The drawing under review shows one solid part. Ordinate dimensions are in mm from its lowest x, y, z. A direction names the side the tool comes from. Give positions to 0.01 mm unless a question says otherwise; leave off trailing zeros. Order: outer loops, then holes, each group sorted by start corner. A loop starts at its lowest first (then second) coordinate and runs counter-clockwise, first axis right, second up. Notation, with made-up numbers: (-22.75, -15) - (13.25, -15) arc R8 ccw to (13.25, -2) - close; hole circle Ø1 at (-36.75, 11.5). An arc over 180 degrees is marked (long way). Use CSV: the item, a comma, the result in double quotes. Start each with the question number.
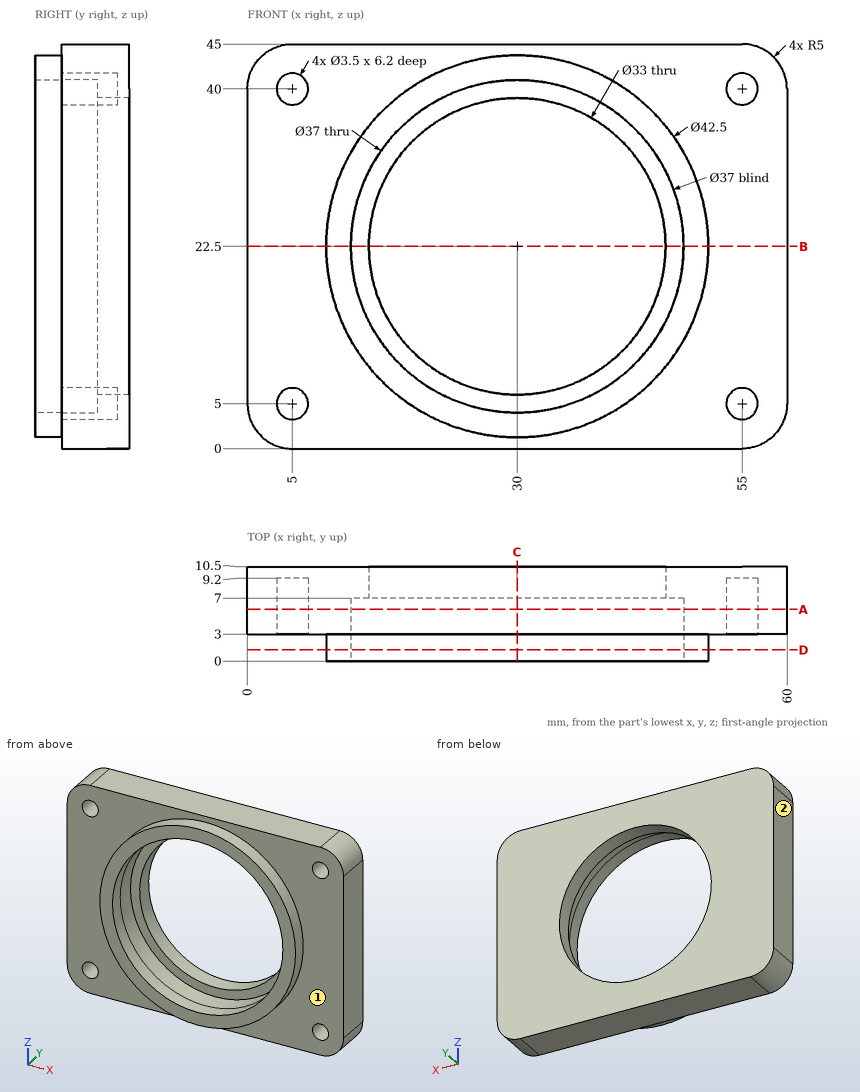
1. Consider section C-C (x = 30). Give the boundary of the cut face in (y, z).
2. To check wall thickness, follow L1, parallel to Z at x = 54, y = 7.5; L2, parallel to X at y = 5.55, z = 22.5; L3, parallel to Z at x = 30, y = 4.15. State the ranges of each line that lie inside material, in increasing order. Write a range as [from, to].
3. Clearance check with flat-ended pins moving along their axes: pin 1 (4 mm diameter, centred on y = 5.5, z = 11.5, fed in from -X); pin 2 (1.8 mm diameter, centred on x = 54, z = 40.5, fed in from -Y); pin 3 (2 mm diameter, centred on x = 55, z = 40, fed in from -Y); pin 4 (22 mm diameter, centred on x = 30, z = 22.5, fed in from -Y). State where each tip first meets the part, or that it passes through.
4. Consider section A-A (y = 5.75). Give the boundary of the cut face in (x, z), and give its area (3 significant figures).
5. Tool access review of the marked faces 1 and 2: name each direction out of +Z, -Z, +X, -X, +Y, -Y from which nothing blocks a thin tool from reaching the whole face with its end or side.
6. Consider section B-B (z = 22.5). Give the boundary of the cut face in (x, y).
7. Consider section D-D (y = 1.25). Give the boundary of the cut face in (x, z).
Answers follow:
1,outline,"(0, 1.25) - (3, 1.25) - (3, 0) - (10.5, 0) - (10.5, 6) - (7, 6) - (7, 4) - (0, 4) - close; (0, 41) - (7, 41) - (7, 39) - (10.5, 39) - (10.5, 45) - (3, 45) - (3, 43.75) - (0, 43.75) - close"
2,L1,"z = [0, 3.56], [6.44, 38.56], [41.44, 45]"
2,L2,"x = [0, 11.5], [48.5, 60]"
2,L3,"z = [0, 4], [41, 45]"
3,pin 1,"stops at x = 0"
3,pin 2,"stops at y = 3"
3,pin 3,"stops at y = 9.2"
3,pin 4,"passes through"
4,outline,"(0, 5) arc R5 ccw to (5, 0) - (55, 0) arc R5 ccw to (60, 5) - (60, 40) arc R5 ccw to (55, 45) - (5, 45) arc R5 ccw to (0, 40) - close; hole circle Ø3.5 at (5, 5); hole circle Ø3.5 at (5, 40); hole circle Ø37 at (30, 22.5); hole circle Ø3.5 at (55, 5); hole circle Ø3.5 at (55, 40)"
4,area,"1,560 mm^2"
5,face 1,"-Y"
5,face 2,"+Z, -Z, -X, +Y, -Y"
6,outline,"(0, 3) - (8.75, 3) - (8.75, 0) - (11.5, 0) - (11.5, 7) - (13.5, 7) - (13.5, 10.5) - (0, 10.5) - close; (46.5, 7) - (48.5, 7) - (48.5, 0) - (51.25, 0) - (51.25, 3) - (60, 3) - (60, 10.5) - (46.5, 10.5) - close"
7,outline,"circle Ø42.5 at (30, 22.5); hole circle Ø37 at (30, 22.5)"
